Input: part model. Units: mm. Frame: model coordinates. A direction names the side the tool comes from. Coordinates: 2 decimals unless noted, no trailing zeros. Write each loop counter-clockwise with the first axis right and the second up, starting at its lowest first coordinate (ties: lowest second). Pieces come first, ordered by that corner, then holes. Notation, with made-up numbers: (36, 87) - (60, 87) arc R27 ccw to (60, 114) - close; hole circle Ø10 at (17.5, 34.5). An arc over 180 degrees is marked (long way). Use a Markdown table: item, result. Add a question column.
Q1. Set-up query: faces 1 (the face through (-39.71, 202.889, -41.734)), 2 (the face through (37.305, -1.61, 0.14)), 3 (the face through (-8, 0, -1)). Return all of +Z, -Z, +X, -X, +Y, -Y with unobstructed straight access to the full face (end or side cutting, diameter ignored); none if empty.
Q2. Section query D-D (z = -21.5). Return the cut outline in (x, y) (1 decimal).
Q3. Pin query (flat end, axial travel): P1, Ø23, axis at y = 33.34, z = 0, coming from the +X side; P2, Ø3.5, axis at y = -1, z = -36, coming from the +X side; P3, Ø10, axis at x = 1.5, z = 0, coming from the +Y side; P4, Ø4, axis at y = 92.5, z = 33.5, coming from the +X side. Return the tip coordinate at first contact, or that it passes through.
Q4. Section query B-B (x = 0). Return the cut outline in (y, z) (3 decimals), then the cut area to 3 significant figures.
Q5. Material intervals for probe 1 along Z at (x, y) = (0, -1.3); probe 2 along Y at (x, z) = (-16.5, -10) (3 decimals); probe 3 along X at (y, z) = (162.5, -40.5) (3 decimals), sorted ascending. Write a range as from..to.
Q6. Section query C-C (z = 0). Return the cut outline in (x, y) (1 decimal).
Q7. Section query A-A (y = 186). Return the cut outline in (x, z) (3 decimals).
Q8. Mould query, pull axis X, two halves, no side actions, for faces 4 (the face through (-41.275, 106, 1)), 5 (the face through (2.564, -1.61, -52.554)), 6 (the face through (-8, -3.175, -1)). Classes: released by +X, released by -X, zero draft, split by the parting line, or undercut.
from build123d import *

# Parameters (mm, degrees)
EXTRUDE1_DEPTH             = 63.5
EXTRUDE1_DEPTH_BACK        = 63.5
CUT_EXTRUDE2_REACH         = 230.798
SKETCH2_R                  = 5.55625
EXTRUDE2_DEPTH             = 3.175
CUT_EXTRUDE3_REACH         = 237.498
SKETCH4_R                  = 12.7
CUT_EXTRUDE4_DEPTH         = 236.497746224
FILLET1_R                  = 9.525
CUT_EXTRUDE7_REACH         = 237.498
FLATTEN_BENDS1_OUTLINE_W   = 4.987278338
FLATTEN_BENDS1_OUTLINE_H   = 127
FLATTEN_BENDS1_DEPTH       = 212.725
FLATTEN_BENDS1_START       = -3.175
FLATTEN_BENDS1_2_OUTLINE_R = 12.7
FLATTEN_BENDS1_2_DEPTH     = 3.175
PROCESS_BENDS1_START       = -252.637278338
PROCESS_BENDS1_OUTLINE_W   = 3.175
PROCESS_BENDS1_OUTLINE_H   = 127
PROCESS_BENDS1_DEPTH       = 211.622562692
PROCESS_BENDS1_START_2     = -41.275
PROCESS_BENDS1_2_OUTLINE_W = 3.175
PROCESS_BENDS1_2_OUTLINE_H = 6.35
PROCESS_BENDS1_2_DEPTH     = 0.287614639
PROCESS_BENDS1_START_3     = -40.987385361
PROCESS_BENDS1_3_OUTLINE_R = 12.7
PROCESS_BENDS1_3_DEPTH     = 2.887385361
PROCESS_BENDS1_4_OUTLINE_R = 12.7
PROCESS_BENDS1_4_DEPTH     = 4.7625
PROCESS_BENDS1_START_4     = -64
PROCESS_BENDS1_5_DEPTH     = 128
PROCESS_BENDS1_START_5     = -47.625
PROCESS_BENDS1_6_DEPTH     = 95.25


with BuildPart() as part:
    # Sketch1 → Extrude1 (new, two sides: drawn at the far end of the back side and taken through both)
    with BuildSketch(Plane.XY.offset(-EXTRUDE1_DEPTH_BACK)):
        with BuildLine():
            Line((18.25625, 0), (-36.5125, 0))
            ThreePointArc((-36.5125, 0), (-37.635032015, 0.464967985), (-38.1, 1.5875))
            Line((-38.1, 1.5875), (-38.1, 212.725))
            Line((-38.1, 212.725), (-41.275, 212.725))
            Line((-41.275, 212.725), (-41.275, 1.5875))
            ThreePointArc((-41.275, 1.5875), (-39.880096045, -1.780096045), (-36.5125, -3.175))
            Line((-36.5125, -3.175), (18.25625, -3.175))
            Line((18.25625, -3.175), (18.25625, 0))
        make_face()
    extrude(amount=EXTRUDE1_DEPTH + EXTRUDE1_DEPTH_BACK)

    # Sketch2 → Cut-Extrude2 (cut, up to next)
    with BuildSketch(Plane.XZ.offset(3.175), mode=Mode.PRIVATE) as cut_extrude2_sk1:
        with Locations((0, -47.625)):
            Circle(SKETCH2_R)
    cut_extrude2_tool1 = extrude(cut_extrude2_sk1.sketch, amount=-CUT_EXTRUDE2_REACH, mode=Mode.PRIVATE) & part.part
    # Sketch2 → Cut-Extrude2 (cut, up to next)
    with BuildSketch(Plane.XZ.offset(3.175), mode=Mode.PRIVATE) as cut_extrude2_sk2:
        with Locations((0, 47.625)):
            Circle(SKETCH2_R)
    cut_extrude2_tool2 = extrude(cut_extrude2_sk2.sketch, amount=-CUT_EXTRUDE2_REACH, mode=Mode.PRIVATE) & part.part
    add(cut_extrude2_tool1.solids().sort_by_distance((0, -3.175, -47.625))[0], mode=Mode.SUBTRACT)
    add(cut_extrude2_tool2.solids().sort_by_distance((0, -3.175, 47.625))[0], mode=Mode.SUBTRACT)

    # Sketch3 → Extrude2 (add)
    with BuildSketch(Plane.XZ.offset(3.175)):
        with BuildLine():
            Line((18.25625, -19.05), (18.25625, 19.05))
            ThreePointArc((18.25625, 19.05), (21.975993879, 10.069743879), (30.95625, 6.35))
            ThreePointArc((30.95625, 6.35), (37.30625, 0), (30.95625, -6.35))
            ThreePointArc((30.95625, -6.35), (21.975993879, -10.069743879), (18.25625, -19.05))
        make_face()
    extrude(amount=-EXTRUDE2_DEPTH)

    # Sketch4 → Cut-Extrude3 (cut, up to next)
    with BuildSketch(Plane.ZY.offset(41.275), mode=Mode.PRIVATE) as cut_extrude3_sk1:
        with Locations((0, 33.3375)):
            Circle(SKETCH4_R)
    cut_extrude3_tool1 = extrude(cut_extrude3_sk1.sketch, amount=-CUT_EXTRUDE3_REACH, mode=Mode.PRIVATE) & part.part
    add(cut_extrude3_tool1.solids().sort_by_distance((-41.275, 33.3375, 0))[0], mode=Mode.SUBTRACT)

    # Sketch5 → Cut-Extrude4 (cut, through all)
    with BuildSketch(Plane.ZY.offset(41.275)):
        Polygon((44.45, 705.492076342), (44.45, 212.725), (44.45, 200.025), (-44.45, 200.025), (-44.45, 212.725), (-44.45, 705.492076342), (-44.45, 1691.026229027), (44.45, 1691.026229027), align=None)
    extrude(amount=-CUT_EXTRUDE4_DEPTH, mode=Mode.SUBTRACT)

    # Fillet1
    fillet1_edges = [part.edges().sort_by_distance(p)[0] for p in [
        (-39.6875, 200.025, 44.45),
        (-39.6875, 200.025, -44.45),
    ]]
    fillet(fillet1_edges, radius=FILLET1_R)

    # Sketch6 → Cut-Extrude7 (cut, up to next)
    with BuildSketch(Plane.ZY.offset(41.275), mode=Mode.PRIVATE) as cut_extrude7_sk1:
        with BuildLine():
            Line((-47.625, 192.151), (-47.625, 173.101))
            ThreePointArc((-47.625, 173.101), (-44.45, 169.926), (-41.275, 173.101))
            Line((-41.275, 173.101), (-41.275, 192.151))
            ThreePointArc((-41.275, 192.151), (-44.45, 195.326), (-47.625, 192.151))
        make_face()
    cut_extrude7_tool1 = extrude(cut_extrude7_sk1.sketch, amount=-CUT_EXTRUDE7_REACH, mode=Mode.PRIVATE) & part.part
    # Sketch6 → Cut-Extrude7 (cut, up to next)
    with BuildSketch(Plane.ZY.offset(41.275), mode=Mode.PRIVATE) as cut_extrude7_sk2:
        with BuildLine():
            Line((47.625, 173.101), (47.625, 192.151))
            ThreePointArc((47.625, 192.151), (44.45, 195.326), (41.275, 192.151))
            Line((41.275, 192.151), (41.275, 173.101))
            ThreePointArc((41.275, 173.101), (44.45, 169.926), (47.625, 173.101))
        make_face()
    cut_extrude7_tool2 = extrude(cut_extrude7_sk2.sketch, amount=-CUT_EXTRUDE7_REACH, mode=Mode.PRIVATE) & part.part
    add(cut_extrude7_tool1.solids().sort_by_distance((-41.275, 182.626, -44.45))[0], mode=Mode.SUBTRACT)
    add(cut_extrude7_tool2.solids().sort_by_distance((-41.275, 182.626, 44.45))[0], mode=Mode.SUBTRACT)

    # Flatten-Bends1: read off the stored shape, not the designer's step
    # Flatten-Bends1 outline → Flatten-Bends1 (cut)
    with BuildSketch(Plane(origin=(0, 0, 0), x_dir=(1, 0, 0), z_dir=(0, 1, 0))):
        with Locations((-39.006139169, 0)):
            Rectangle(FLATTEN_BENDS1_OUTLINE_W, FLATTEN_BENDS1_OUTLINE_H)
    extrude(amount=FLATTEN_BENDS1_DEPTH, mode=Mode.SUBTRACT)

    # Flatten-Bends1 2 outline → Flatten-Bends1 2 (add)
    with BuildSketch(Plane(origin=(0, 0, 0), x_dir=(1, 0, 0), z_dir=(0, 1, 0)).offset(FLATTEN_BENDS1_START)):
        with BuildLine():
            Line((-252.637278338, -44.45), (-252.637278338, -63.5))
            Line((-252.637278338, -63.5), (-36.5125, -63.5))
            Line((-36.5125, -63.5), (-36.5125, 63.5))
            Line((-36.5125, 63.5), (-252.637278338, 63.5))
            Line((-252.637278338, 63.5), (-252.637278338, 44.45))
            Line((-252.637278338, 44.45), (-249.462278338, 44.45))
            ThreePointArc((-249.462278338, 44.45), (-242.727086247, 41.660192091), (-239.937278338, 34.925))
            Line((-239.937278338, 34.925), (-239.937278338, -34.925))
            ThreePointArc((-239.937278338, -34.925), (-242.727086247, -41.660192091), (-249.462278338, -44.45))
            Line((-249.462278338, -44.45), (-252.637278338, -44.45))
        make_face()
        with BuildLine():
            Line((-213.013278338, -47.625), (-232.063278338, -47.625))
            ThreePointArc((-232.063278338, -47.625), (-235.238278338, -44.45), (-232.063278338, -41.275))
            Line((-232.063278338, -41.275), (-213.013278338, -41.275))
            ThreePointArc((-213.013278338, -41.275), (-209.838278338, -44.45), (-213.013278338, -47.625))
        make_face(mode=Mode.SUBTRACT)
        with Locations((-73.249778338, 0)):
            Circle(FLATTEN_BENDS1_2_OUTLINE_R, mode=Mode.SUBTRACT)
        with BuildLine():
            Line((-232.063278338, 47.625), (-213.013278338, 47.625))
            ThreePointArc((-213.013278338, 47.625), (-209.838278338, 44.45), (-213.013278338, 41.275))
            Line((-213.013278338, 41.275), (-232.063278338, 41.275))
            ThreePointArc((-232.063278338, 41.275), (-235.238278338, 44.45), (-232.063278338, 47.625))
        make_face(mode=Mode.SUBTRACT)
    extrude(amount=FLATTEN_BENDS1_2_DEPTH)

    # Process-Bends1: read off the stored shape, not the designer's step
    # Process-Bends1 outline → Process-Bends1 (cut)
    with BuildSketch(Plane.YZ.offset(PROCESS_BENDS1_START)):
        with Locations((-1.5875, 0)):
            Rectangle(PROCESS_BENDS1_OUTLINE_W, PROCESS_BENDS1_OUTLINE_H)
    extrude(amount=PROCESS_BENDS1_DEPTH, mode=Mode.SUBTRACT)

    # Process-Bends1 2 outline → Process-Bends1 2 (cut)
    with BuildSketch(Plane.YZ.offset(PROCESS_BENDS1_START_2)):
        with Locations((-1.5875, -44.45)):
            Rectangle(PROCESS_BENDS1_2_OUTLINE_W, PROCESS_BENDS1_2_OUTLINE_H)
        with Locations((-1.5875, 44.45)):
            Rectangle(PROCESS_BENDS1_2_OUTLINE_W, PROCESS_BENDS1_2_OUTLINE_H)
    extrude(amount=PROCESS_BENDS1_2_DEPTH, mode=Mode.SUBTRACT)

    # Process-Bends1 3 outline → Process-Bends1 3 (add)
    with BuildSketch(Plane.YZ.offset(PROCESS_BENDS1_START_3)):
        with BuildLine():
            Line((212.725, -44.45), (209.55, -44.45))
            ThreePointArc((209.55, -44.45), (202.814807909, -41.660192091), (200.025, -34.925))
            Line((200.025, -34.925), (200.025, 34.925))
            ThreePointArc((200.025, 34.925), (202.814807909, 41.660192091), (209.55, 44.45))
            Line((209.55, 44.45), (212.725, 44.45))
            Line((212.725, 44.45), (212.725, 63.5))
            Line((212.725, 63.5), (0, 63.5))
            Line((0, 63.5), (0, -63.5))
            Line((0, -63.5), (212.725, -63.5))
            Line((212.725, -63.5), (212.725, -44.45))
        make_face()
        with BuildLine():
            Line((192.151, -47.625), (173.101, -47.625))
            ThreePointArc((173.101, -47.625), (169.926, -44.45), (173.101, -41.275))
            Line((173.101, -41.275), (192.151, -41.275))
            ThreePointArc((192.151, -41.275), (195.326, -44.45), (192.151, -47.625))
        make_face(mode=Mode.SUBTRACT)
        with Locations((33.3375, 0)):
            Circle(PROCESS_BENDS1_3_OUTLINE_R, mode=Mode.SUBTRACT)
        with BuildLine():
            Line((192.151, 41.275), (173.101, 41.275))
            ThreePointArc((173.101, 41.275), (169.926, 44.45), (173.101, 47.625))
            Line((173.101, 47.625), (192.151, 47.625))
            ThreePointArc((192.151, 47.625), (195.326, 44.45), (192.151, 41.275))
        make_face(mode=Mode.SUBTRACT)
    extrude(amount=PROCESS_BENDS1_3_DEPTH)

    # Process-Bends1 4 outline → Process-Bends1 4 (add)
    with BuildSketch(Plane.YZ.offset(PROCESS_BENDS1_START_2)):
        with BuildLine():
            Line((212.725, 63.5), (0, 63.5))
            Line((0, 63.5), (0, -63.5))
            Line((0, -63.5), (212.725, -63.5))
            Line((212.725, -63.5), (212.725, -44.45))
            Line((212.725, -44.45), (209.55, -44.45))
            ThreePointArc((209.55, -44.45), (202.814807909, -41.660192091), (200.025, -34.925))
            Line((200.025, -34.925), (200.025, 34.925))
            ThreePointArc((200.025, 34.925), (202.814807909, 41.660192091), (209.55, 44.45))
            Line((209.55, 44.45), (212.725, 44.45))
            Line((212.725, 44.45), (212.725, 63.5))
        make_face()
        with BuildLine():
            Line((192.151, -47.625), (173.101, -47.625))
            ThreePointArc((173.101, -47.625), (169.926, -44.45), (173.101, -41.275))
            Line((173.101, -41.275), (192.151, -41.275))
            ThreePointArc((192.151, -41.275), (195.326, -44.45), (192.151, -47.625))
        make_face(mode=Mode.SUBTRACT)
        with Locations((33.3375, 0)):
            Circle(PROCESS_BENDS1_4_OUTLINE_R, mode=Mode.SUBTRACT)
        with BuildLine():
            Line((192.151, 41.275), (173.101, 41.275))
            ThreePointArc((173.101, 41.275), (169.926, 44.45), (173.101, 47.625))
            Line((173.101, 47.625), (192.151, 47.625))
            ThreePointArc((192.151, 47.625), (195.326, 44.45), (192.151, 41.275))
        make_face(mode=Mode.SUBTRACT)
    extrude(amount=PROCESS_BENDS1_4_DEPTH)

    # Process-Bends1 5 outline → Process-Bends1 5 (cut)
    with BuildSketch(Plane.XY.offset(PROCESS_BENDS1_START_4)):
        with BuildLine():
            Line((-36.5125, 212.725), (-38.1, 212.725))
            Line((-38.1, 212.725), (-38.1, 1.5875))
            ThreePointArc((-38.1, 1.5875), (-37.635032015, 0.464967985), (-36.5125, 0))
            Line((-36.5125, 0), (-36.5125, 212.725))
        make_face()
        with BuildLine():
            Line((-41.275, 1.5875), (-41.275, 0))
            Line((-41.275, 0), (-41.014715646, 0))
            Line((-41.014715646, 0), (-41.014715646, -3.175))
            Line((-41.014715646, -3.175), (-36.5125, -3.175))
            ThreePointArc((-36.5125, -3.175), (-39.880096045, -1.780096045), (-41.275, 1.5875))
        make_face()
    extrude(amount=PROCESS_BENDS1_5_DEPTH, mode=Mode.SUBTRACT)

    # Process-Bends1 6 outline → Process-Bends1 6 (add)
    with BuildSketch(Plane.XY.offset(PROCESS_BENDS1_START_5)):
        with BuildLine():
            Line((-40.987385361, 0), (-41.00262806, 0))
            ThreePointArc((-41.00262806, 0), (-40.995057012, -0.021253828), (-40.987385361, -0.04247155))
            Line((-40.987385361, -0.04247155), (-40.987385361, 0))
        make_face()
    extrude(amount=PROCESS_BENDS1_6_DEPTH)


solid = part.part
Values follow:
| question | item | result |
|---|---|---|
| 1 | face 1 | +X, -X, +Y |
| 1 | face 2 | +X, +Y, -Y |
| 1 | face 3 | +Z, -Z, +X, +Y |
| 2 | outline | (-41.3, 1.6) arc R4.8 ccw to (-36.5, -3.2) - (18.3, -3.2) - (18.3, 0) - (-36.5, 0) arc R1.6 cw to (-38.1, 1.6) - (-38.1, 200) - (-41.3, 200) - close |
| 3 | P1 | through |
| 3 | P2 | x = 18.26 |
| 3 | P3 | y = 0 |
| 3 | P4 | x = -38.1 |
| 4 | outline | (-3.175, -63.5) - (0, -63.5) - (0, -53.181) - (-3.175, -53.181) - close; (-3.175, -42.069) - (0, -42.069) - (0, 42.069) - (-3.175, 42.069) - close; (-3.175, 53.181) - (0, 53.181) - (0, 63.5) - (-3.175, 63.5) - close |
| 4 | area | 333 mm2 |
| 5 | probe 1 | -63.5..-53.18, -42.07..42.07, 53.18..63.5 |
| 5 | probe 2 | -3.175..0 |
| 5 | probe 3 | -41.275..-38.1 |
| 6 | outline | (-41.3, 1.6) arc R4.8 ccw to (-36.5, -3.2) - (37.3, -3.2) - (37.3, 0) - (-36.5, 0) arc R1.6 cw to (-38.1, 1.6) - (-38.1, 20.6) - (-41.3, 20.6) - close; (-41.3, 46) - (-38.1, 46) - (-38.1, 200) - (-41.3, 200) - close |
| 7 | outline | (-41.275, -63.5) - (-38.1, -63.5) - (-38.1, -47.625) - (-41.275, -47.625) - close; (-41.275, -41.275) - (-38.1, -41.275) - (-38.1, 41.275) - (-41.275, 41.275) - close; (-41.275, 47.625) - (-38.1, 47.625) - (-38.1, 63.5) - (-41.275, 63.5) - close |
| 8 | face 4 | released by -X |
| 8 | face 5 | undercut |
| 8 | face 6 | zero draft |
